Design review of the part built by this model. Coordinates are the model's own, in mm. A direction names the side the tool comes from. Coordinates: 2 decimals unless noted, no trailing zeros. Order: outer loops, then holes, each group sorted by start corner. A loop starts at its lowest first (then second) coordinate and runs counter-clockwise, first axis right, second up. Notation, with made-up numbers: (46, 15) -> (69, 15) arc R36 ccw to (69, 53) -> close; hole circle Ø1 at (-15, 8.25). An arc over 180 degrees is marked (long way). Use a Markdown table: item, result. Add a question column.
Q1. Add section B-B (z = -5). State the section outline as (x, y) points, then the cut area to 3 significant figures.
Q2. Add section A-A (y = 3.75). State the section outline as (x, z) points, then the cut area to 3 significant figures.
Q3. Machinability: for faces 5 (the face through (26, 1, 31)), 6 (the face through (-26, 1, 31)), 7 (the face through (26, 1, -31)), 8 (the face through (0, 5, 32)), which of the approach directions +Z, -Z, +X, -X, +Y, -Y give a long, thin tool a straight path to every point of the face, cutting with its end or side? Answer none if there is none.
Q4. The part is to be moulded in two halves that separate along X. For faces 1 (the face through (-30, 4, 0)), 2 (the face through (0, 4, 35)), 3 (the face through (30, 4, 0)), 4 (the face through (0, 1, -13)), say which applies: pulls with the +X half, pulls with the -X half, needs draft (parallel to the pull), parting line crosses it, or undercut.
Q5. Add section D-D (x = 21). State the section outline as (y, z) points, then the cut area to 3 significant figures.
Q6. Add section C-C (x = 8.5). State the section outline as (y, z) points, then the cut area to 3 significant figures.
Q7. Insertion check: pin 1 (3 mm diameter, centred on x = 11, z = 1, fed in from +Y); pin 2 (0.5 mm diameter, centred on y = 0.5, z = 32.5, fed in from +X); pin 3 (0.5 mm diameter, centred on x = -26, y = 0.5, fed in from +Z); pin 4 (1 mm diameter, centred on x = 22, z = -19, fed in from -Y). Each pin has a flat end and moves straight along its axis. Give the tip position at first contact, or say it passes through.
Q8. Wall thickness on probe 1 along X at (y, z) = (4.5, 30); probe 2 along Z at (x, y) = (15, 2.75); probe 3 along Y at (x, z) = (2, -31): over which ranges is each line inside the solid? List them lowest first.
Autodesk Inventor part; units mm, degrees
ref_plane "YZ Plane" through (0, 0, 0) normal (1, 0, 0) x (0, 1, 0)
ref_plane "XZ Plane" through (0, 0, 0) normal (0, 1, 0) x (-1, 0, 0)
ref_plane "XY Plane" through (0, 0, 0) normal (0, 0, 1) x (1, 0, 0)
sketch "Sketch1" plane through (0, 0, 0) normal (0, 1, 0) x (-1, 0, 0)
  line L0 (-30, 35) -> (30, 35)
  line L1 (30, 35) -> (30, -35)
  line L2 (30, -35) -> (-30, -35)
  line L3 (-30, -35) -> (-30, 35)
  line L4 (-30, 35) -> (30, -35) construction
  line L5 (30, 35) -> (-30, -35) construction
  point P0 (0, 0)
  dimension "d0" = 60
  dimension "d1" = 70
extrude "Extrusion1" add sketch "Sketch1" along normal blind 8
sketch "Sketch2" plane through (0, 8, 0) normal (0, 1, 0) x (1, 0, 0)
  line L0 (27, -32) -> (27, 32)
  line L1 (27, 32) -> (-27, 32)
  line L2 (-27, 32) -> (-27, -32)
  line L3 (-27, -32) -> (27, -32)
  line L4 (27, -32) -> (-27, 32) construction
  line L5 (27, 32) -> (-27, -32) construction
  point P0 (0, 0)
  dimension "d4" = 64
  dimension "d5" = 54
extrude "Extrusion2" cut sketch "Sketch2" against normal blind 6
sketch "Sketch3" plane through (0, 2, 0) normal (0, 1, 0) x (1, 0, 0)
  line L0 (-12, -12) -> (12, -12)
  line L1 (12, -12) -> (12, 12)
  line L2 (12, 12) -> (-12, 12)
  line L3 (-12, 12) -> (-12, -12)
  line L4 (-12, -12) -> (12, 12) construction
  line L5 (12, -12) -> (-12, 12) construction
  line L6 (-13, -13) -> (13, -13)
  line L7 (13, -13) -> (13, 13)
  line L8 (13, 13) -> (-13, 13)
  line L9 (-13, 13) -> (-13, -13)
  line L10 (-13, -13) -> (13, 13) construction
  line L11 (13, -13) -> (-13, 13) construction
  circle A0 centre (-13, -13) radius 1.5
  circle A1 centre (-13, 13) radius 1.5
  circle A2 centre (13, 13) radius 1.5
  circle A3 centre (13, -13) radius 1.5
  point P0 (0, 0)
  dimension "d8" = 24
  dimension "d9" = 24
  dimension "d10" = 26
  dimension "d11" = 26
  dimension "d23" = 3
  dimension "d24" = 3
  dimension "d25" = 3
  dimension "d26" = 3
extrude "Extrusion3" cut sketch "Sketch3" against normal blind 1.5
sketch "Sketch4" plane through (0, 0.5, 0) normal (0, 1, 0) x (1, 0, 0)
  line L0 (-12, -12) -> (12, -12)
  line L1 (12, -12) -> (12, 12)
  line L2 (12, 12) -> (-12, 12)
  line L3 (-12, 12) -> (-12, -12)
  line L4 (-12, -12) -> (12, 12) construction
  line L5 (12, -12) -> (-12, 12) construction
  point P0 (0, 0)
  dimension "d18" = 24
  dimension "d19" = 24
extrude "Extrusion4" cut sketch "Sketch4" against normal up to next
sketch "Sketch5" plane through (0, 2, 0) normal (0, 1, 0) x (1, 0, 0)
  point P0 (0, 0)
sketch "Sketch6" plane through (0, 2, 0) normal (0, 1, 0) x (1, 0, 0)
  line L0 (20, 34) -> (-20, 34)
  line L1 (-20, 34) -> (-20, -6)
  line L2 (-20, -6) -> (20, -6)
  line L3 (20, -6) -> (20, 34)
  line L4 (20, 34) -> (-20, -6) construction
  line L5 (-20, 34) -> (20, -6) construction
  line L6 (12, -12) -> (-12, -12)
  point P0 (0, 0)
  point P1 (0, 14)
  dimension "d27" = 40
  dimension "d28" = 40
  dimension "d29" = 6
sketch "Sketch7" plane through (0, 8, 0) normal (0, 1, 0) x (1, 0, 0)
  point P0 (0, 0)
sketch "Sketch8" plane through (0, 0, 0) normal (0, -1, 0) x (1, 0, 0)
  line L0 (-30, -35) -> (-30, 35)
  line L1 (-30, -35) -> (-22, -35)
  line L2 (-22, -35) -> (-22, -27)
  line L3 (-22, -27) -> (-30, -27)
  line L4 (-30, -27) -> (-30, -35)
  line L5 (-30, 35) -> (30, 35)
  line L6 (-30, 35) -> (-22, 35)
  line L7 (-22, 35) -> (-22, 27)
  line L8 (-22, 27) -> (-30, 27)
  line L9 (-30, 27) -> (-30, 35)
  line L10 (30, -35) -> (30, 35)
  line L11 (30, 35) -> (22, 35)
  line L12 (22, 35) -> (22, 27)
  line L13 (22, 27) -> (30, 27)
  line L14 (30, 27) -> (30, 35)
  line L15 (30, -35) -> (22, -35)
  line L16 (22, -35) -> (22, -27)
  line L17 (22, -27) -> (30, -27)
  line L18 (30, -27) -> (30, -35)
  point P0 (0, 0)
  dimension "d30" = 8
  dimension "d31" = 8
  dimension "d32" = 8
  dimension "d33" = 8
  dimension "d34" = 8
  dimension "d35" = 8
  dimension "d36" = 8
  dimension "d37" = 8
extrude "Extrusion5" cut sketch "Sketch8" against normal blind 1
sketch "Sketch9" plane through (0, 8, 0) normal (0, 1, 0) x (1, 0, 0)
  line L0 (30, 35) -> (22, 35)
  line L1 (22, 35) -> (22, 27)
  line L2 (30, 35) -> (22, 35)
  line L3 (22, 35) -> (22, 27)
  line L4 (22, 27) -> (30, 27)
  line L5 (30, 27) -> (30, 35)
  circle A0 centre (26, 31) radius 5.5
  point P0 (0, 0)
  dimension "d40" = 11
properties part number "base"
Established:
| question | item | result |
|---|---|---|
| 1 | outline | (-30, 0) -> (-12, 0) -> (-12, 0.5) -> (-13, 0.5) -> (-13, 2) -> (-27, 2) -> (-27, 8) -> (-30, 8) -> close; (12, 0) -> (30, 0) -> (30, 8) -> (27, 8) -> (27, 2) -> (13, 2) -> (13, 0.5) -> (12, 0.5) -> close |
| 1 | area | 105 mm^2 |
| 2 | outline | (-30, -35) -> (30, -35) -> (30, 35) -> (-30, 35) -> close; hole (-27, -32) -> (27, -32) -> (27, 32) -> (-27, 32) -> close |
| 2 | area | 744 mm^2 |
| 3 | face 5 | +Z, +X, -Y |
| 3 | face 6 | +Z, -X, -Y |
| 3 | face 7 | -Z, +X, -Y |
| 3 | face 8 | +Y |
| 4 | face 1 | pulls with the -X half |
| 4 | face 2 | needs draft |
| 4 | face 3 | pulls with the +X half |
| 4 | face 4 | undercut |
| 5 | outline | (0, -35) -> (8, -35) -> (8, -32) -> (2, -32) -> (2, 32) -> (8, 32) -> (8, 35) -> (0, 35) -> close |
| 5 | area | 176 mm^2 |
| 6 | outline | (0, -35) -> (8, -35) -> (8, -32) -> (2, -32) -> (2, -13) -> (0.5, -13) -> (0.5, -12) -> (0, -12) -> close; (0, 12) -> (0.5, 12) -> (0.5, 13) -> (2, 13) -> (2, 32) -> (8, 32) -> (8, 35) -> (0, 35) -> close |
| 6 | area | 125 mm^2 |
| 7 | pin 1 | y = 0.5 |
| 7 | pin 2 | x = 22 |
| 7 | pin 3 | z = 27 |
| 7 | pin 4 | y = 0 |
| 8 | probe 1 | -30 to -27, 27 to 30 |
| 8 | probe 2 | -35 to -32, 32 to 35 |
| 8 | probe 3 | 0 to 2 |
